```python
from build123d import *

# Parameters (mm, degrees)
SKETCH1_R           = 1.75
BOSS_EXTRUDE1_DEPTH = 5


with BuildPart() as part:
    # Sketch1 → Boss-Extrude1 (new body)
    with BuildSketch(Plane.XY):
        with BuildLine():
            Line((0, 4), (11.455291715, 4))
            Line((11.455291715, 4), (50.906715776, 10.601904234))
            Line((50.906715776, 10.601904234), (54.065764272, 9.095115396))
            Line((54.065764272, 9.095115396), (49.519627933, 3.772273636))
            ThreePointArc((49.519627933, 3.772273636), (41.094269374, 3.768555825), (34, -0.776553935))
            ThreePointArc((34, -0.776553935), (27.921587079, -2.096367305), (22, -4))
            Line((22, -4), (0, -4))
            ThreePointArc((0, -4), (-4, 0), (0, 4))
        make_face()
        Circle(SKETCH1_R, mode=Mode.SUBTRACT)
        with Locations((22, 0)):
            Circle(SKETCH1_R, mode=Mode.SUBTRACT)
    extrude(amount=-BOSS_EXTRUDE1_DEPTH)


solid = part.part
```
Source: CAD feature listing. Evaluate the final solid. Frame: model axes, mm. A direction names the side the tool comes from. Coordinates: 2 decimals unless noted, no trailing zeros. Loops run counter-clockwise (first coordinate to the right, second up) from the corner with the lowest first, then second, coordinate; pieces in that order, holes last. Notation, with made-up numbers: M -0.75,39.25 L 6.25,39.25 A27 cw 6.25,59.25 Z; hole C 2.5,89 d3. An arc over 180 degrees is marked long. Use a Markdown table: item, result. Add a question column.
Q1. Section query A-A, the plane z = -3.3. Return loops of the section in (x, y).
Q2. Section query B-B, the plane y = 0. Return loops of the section in (x, z).
Q3. Access query for faces 1 (the cylindrical face through (20.25, 0.08, -2.46)), 2 (the flat face through (6, 4, -2)). Directions: +Z, -Z, +X, -X, +Y, -Y. A direction counts if a zero-diameter tool reaches every point of the face in a straight line with its end or side. Return the directions, or none.
Q4. Section query D-D, the plane x = 26.5. Return loops of the section in (y, z), and give its area (3 significant figures).
Q5. Section query C-C, the plane x = 44. Return loops of the section in (y, z), and give its area (3 significant figures).
Q6. Draft query along X for faces 3 (the flat face through (11, -4, -2)), 4 (the cylindrical face through (1.617, -0.67, -2.465)), 5 (the cylindrical face through (-4, 0, -2)). Return one class per face: pulls with the +X half, pulls with the -X half, needs draft (parallel to the pull), parting line crosses it, or undercut.
Q7. Material intervals for L1, parallel to X at y = 1.5, z = -2.3; L2, parallel to Y at x = 0, z = -2.05; L3, parallel to Y at x = 2.5, z = -1.25, sorted ascending.
Q8. First-contact query: pin 1 (2 mm diameter, centred on x = 0, y = 0, fed in from +Z); pin 2 (3 mm diameter, centred on x = 38.5, z = -4, fed in from +Y); pin 3 (1.5 mm diameter, centred on x = 35, z = -1.5, fed in from -Y); pin 4 (3 mm diameter, centred on x = 34.5, z = -1, fed in from -Y). Flat tips, straight axial feed; report the tip coordinate or a pass-through.
Result:
| question | item | result |
|---|---|---|
| 1 | outline | M 0,-4 L 22,-4 A64 cw 34,-0.78 A15 cw 49.52,3.77 L 54.07,9.1 L 50.91,10.6 L 11.46,4 L 0,4 A4 ccw Z; hole C 0,0 d3.5; hole C 22,0 d3.5 |
| 2 | outline | M -4,-5 L -1.75,-5 L -1.75,0 L -4,0 Z; M 1.75,-5 L 20.25,-5 L 20.25,0 L 1.75,0 Z; M 23.75,-5 L 34.73,-5 L 34.73,0 L 23.75,0 Z |
| 3 | face 1 | +Z, -Z |
| 3 | face 2 | +Z, -Z, -X, +Y |
| 4 | outline | M -2.5,-5 L 6.52,-5 L 6.52,0 L -2.5,0 Z |
| 4 | area | 45.1 mm2 |
| 5 | outline | M 4.32,-5 L 9.45,-5 L 9.45,0 L 4.32,0 Z |
| 5 | area | 25.6 mm2 |
| 6 | face 3 | needs draft |
| 6 | face 4 | undercut |
| 6 | face 5 | pulls with the -X half |
| 7 | L1 | x = -3.71 to -0.9, 0.9 to 21.1, 22.9 to 36.48 |
| 7 | L2 | y = -4 to -1.75, 1.75 to 4 |
| 7 | L3 | y = -4 to 4 |
| 8 | pin 1 | passes through |
| 8 | pin 2 | stops at y = 8.78 |
| 8 | pin 3 | stops at y = -0.5 |
| 8 | pin 4 | stops at y = -0.95 |
